The listing builds one solid part. Answer for the finished solid, in the listing's coordinates (mm). Face numbers are marked on the shaded views. A direction names the side the tool comes from. Round coordinates to 2 decimals unless told otherwise and drop trailing zeros. Write each loop counter-clockwise with the first axis right and the second up, starting at its lowest first coordinate (ties: lowest second). Pieces come first, ordered by that corner, then holes.
from build123d import *

# Parameters (mm, degrees)
BOSS_EXTRUDE1_DEPTH            = 40
SKETCH2_W                      = 40
SKETCH2_H                      = 30
BOSS_EXTRUDE2_DEPTH            = 20
BOSS_EXTRUDE3_DEPTH            = 30
CUT_EXTRUDE1_DEPTH             = 30
SKETCH5_W                      = 70
SKETCH5_H                      = 40
BOSS_EXTRUDE4_DEPTH            = 10
SKETCH6_W                      = 20
SKETCH6_H                      = 20
CUT_EXTRUDE2_DEPTH             = 41
F_10_0_10_DIAMETER_HOLE1_D     = 10
F_10_0_10_DIAMETER_HOLE1_DEPTH = 40
FILLET1_R                      = 20


with BuildPart() as part:
    # Sketch1 → Boss-Extrude1 (new body)
    with BuildSketch(Plane(origin=(0, 0, 0), x_dir=(0, -1, 0), z_dir=(-1, 0, 0))):
        Polygon((-10, -14), (-40, -20), (-10, -20), align=None)
    extrude(amount=-BOSS_EXTRUDE1_DEPTH)

    # Sketch2 → Boss-Extrude2 (add)
    with BuildSketch(Plane(origin=(0, 0, -20), x_dir=(-1, 0, 0), z_dir=(0, 0, -1))):
        with Locations((-20, 25)):
            Rectangle(SKETCH2_W, SKETCH2_H)
    extrude(amount=BOSS_EXTRUDE2_DEPTH)

    # Sketch3 → Boss-Extrude3 (add)
    with BuildSketch(Plane(origin=(40, 0, 0), x_dir=(0, 0, -1), z_dir=(1, 0, 0))):
        Polygon((40, 10), (0, 10), (20, 40), (40, 40), align=None)
    extrude(amount=BOSS_EXTRUDE3_DEPTH)

    # Sketch4 → Cut-Extrude1 (cut)
    with BuildSketch(Plane(origin=(70, 0, 0), x_dir=(0, 0, -1), z_dir=(1, 0, 0))):
        Polygon((20, 40), (0, 10), (30, 10), (30, 30), (40, 30), (40, 40), align=None)
    extrude(amount=-CUT_EXTRUDE1_DEPTH, mode=Mode.SUBTRACT)

    # Sketch5 → Boss-Extrude4 (add)
    with BuildSketch(Plane.XZ.offset(-10)):
        with Locations((35, -20)):
            Rectangle(SKETCH5_W, SKETCH5_H)
    extrude(amount=BOSS_EXTRUDE4_DEPTH)

    # Sketch6 → Cut-Extrude2 (cut, through all)
    with BuildSketch(Plane(origin=(0, 0, -40), x_dir=(-1, 0, 0), z_dir=(0, 0, -1))):
        with Locations((-20, 30)):
            Rectangle(SKETCH6_W, SKETCH6_H)
    extrude(amount=-CUT_EXTRUDE2_DEPTH, mode=Mode.SUBTRACT)

    # Ø10.0 (10) Diameter Hole1
    with Locations(Plane(origin=(0, 0, 0), x_dir=(-1, 0, 0), z_dir=(0, -1, 0))):
        with Locations((-55, 15)):
            Hole(F_10_0_10_DIAMETER_HOLE1_D / 2, depth=F_10_0_10_DIAMETER_HOLE1_DEPTH)

    # Fillet1
    fillet1_edges = [part.edges().sort_by_distance(p)[0] for p in [
        (70, 30, -35),
    ]]
    fillet(fillet1_edges, radius=FILLET1_R)


solid = part.part
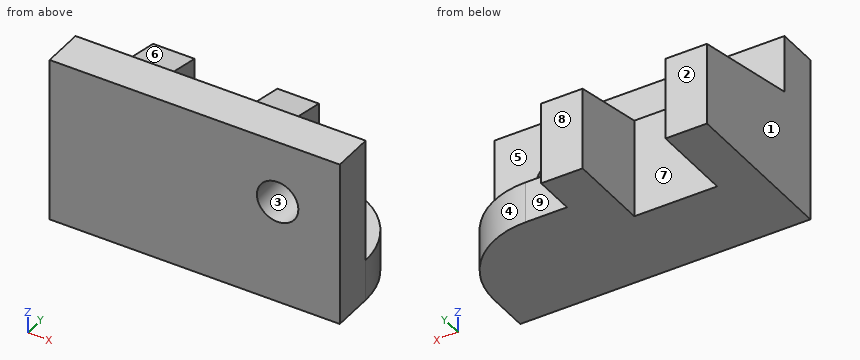
1. Section B-B on z = -15 is taken. Determine the outline of the cut face in (x, y).
Geometry says:
outline: (0, 0) - (50, 0) - (50, 10) - (40, 10) - (40, 15) - (0, 15) - close; (60, 0) - (70, 0) - (70, 10) - (60, 10) - close
2. Section C-C on x = 56.5 is taken. Determine the outline of the cut face in (y, z).
Geometry says:
outline: (0, -40) - (28.91, -40) - (28.91, -30) - (10, -30) - (10, -19.77) - (0, -19.77) - close; (0, -10.23) - (10, -10.23) - (10, 0) - (0, 0) - close
3. Given pin 1 (22 mm diameter, centred on x = 15.5, z = -25.5, fed in from +Y); pin 2 (8 mm diameter, centred on x = 46, z = -33.5, fed in from +Y); pin 3 (6 mm diameter, centred on x = 51, y = 14, fed in from +Z); pin 4 (3 mm diameter, centred on x = 38, y = 22, fed in from +Z), each flat-ended and moving along its own axis, determine where each tip first touches the part or whether it passes through.
Geometry says:
pin 1: stops at y = 40
pin 2: stops at y = 30
pin 3: stops at z = -30
pin 4: stops at z = -16.1
4. Section D-D on x = 46 is taken. Determine the outline of the cut face in (y, z).
Geometry says:
outline: (0, -40) - (30, -40) - (30, -30) - (10, -30) - (10, 0) - (0, 0) - close
5. A tool of negligible diameter and unlimited length cuts with its end or side. For the marked faces 5, 6, 7, 8 and 9, from which of +Z, -Z, +X, -X, +Y, -Y can it reach the whole face along a straight path? Write none if from no direction.
Geometry says:
face 5: +Z, +X, +Y
face 6: +Z, +X, -X, +Y
face 7: +Z, -Z, +Y
face 8: +Z, -Z, +X, -X, +Y
face 9: +Z, -Z, +X, +Y
6. Straight lines are drawn through the part: line 1 along X through (y, z) = (38, -38); line 2 along Z through (x, y) = (55, 4.25); line 3 along Y through (x, z) = (26, -3). For each, find the intervals that lie inside material, in ascending order.
Geometry says:
line 1: x = 0 to 10, 30 to 40
line 2: z = -40 to -20, -10 to 0
line 3: y = 0 to 10
7. For a pull along X with two mould halves and no side action, classify the marked faces 1, 2, 3 and 4 as released by +X, released by -X, zero draft, split by the parting line, or undercut.
Geometry says:
face 1: released by -X
face 2: zero draft
face 3: undercut
face 4: released by +X
8. Section A-A on y = 35.5 is taken. Determine the outline of the cut face in (x, z).
Geometry says:
outline: (0, -40) - (10, -40) - (10, -19.1) - (0, -19.1) - close; (30, -40) - (40, -40) - (40, -19.1) - (30, -19.1) - close
